Can you work these out from the model? Positions are in its coordinate system, mm. Face numbers are marked on the shaded views. A direction names the side the tool comes from. Give positions to 0.01 mm unless a question says otherwise; leave off trailing zeros. Write each loop counter-clockwise with the first axis right and the second up, starting at its lowest first coordinate (ties: lowest second). Pieces come first, ordered by that corner, then holes.
1. Suppose I cut it at B-B (y = 2.2). Please give me the cut outline in (x, z), and give its area (3 significant figures).
2. Thinking about a two-plate mould opening in Z: for the marked faces 4, 5 and 6, which applies, pulls with the +Z half, pulls with the -Z half, needs draft (parallel to the pull), parting line crosses it, or undercut?
3. On a 3-axis mill with a long thin cutter (end or side, diameter ignored), from which of +Z, -Z, +X, -X, +Y, -Y can I reach the whole of each face in a straight line? I mean the marked faces 1, 2 and 3. Say none if no direction works.
4. I'm going to push flat-ended pins straight in: pin 1 (1.3 mm diameter, centred on y = 4, z = -4, fed in from +X); pin 2 (0.6 mm diameter, centred on y = 4, z = -2, fed in from -X). Where does each tip first touch, or does it pass through?
5. Suppose I cut it at A-A (y = 3.75). Please give me the cut outline in (x, z).
6. If I drill on probe 1 along Z at (x, y) = (5, 1.3); probe 2 along Z at (x, y) = (3, 2.75); probe 3 along X at (y, z) = (1.8, -3), over which ranges is the centre line in solid material (lowest first)?
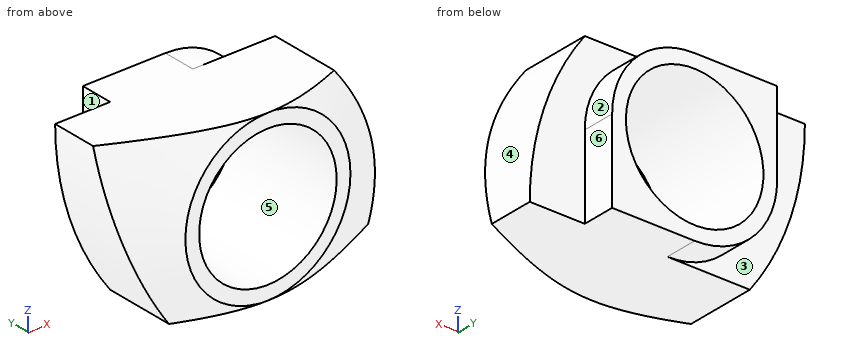
```python
from build123d import *

# Parameters (mm, degrees)
SKETCH_1_W          = 10
SKETCH_1_H          = 6
SKETCH_1_R          = 2.5
EXTRUDE_1_DEPTH     = 3.3
SKETCH_2_R          = 2.5
EXTRUDE_2_DEPTH     = 1.2
CUT_EXTRUDE_1_DEPTH = 5.5


with BuildPart() as part:
    # 草图1 → 凸台-拉伸1 (new body)
    with BuildSketch(Plane(origin=(0, 0, 0), x_dir=(1, 0, 0), z_dir=(0, 1, 0))):
        with Locations((5, 3)):
            Rectangle(SKETCH_1_W, SKETCH_1_H)
        with Locations((5, 3)):
            Circle(SKETCH_1_R, mode=Mode.SUBTRACT)
    extrude(amount=EXTRUDE_1_DEPTH)

    # 草图2 → 凸台-拉伸2 (add)
    with BuildSketch(Plane(origin=(0, 3.3, 0), x_dir=(1, 0, 0), z_dir=(0, 1, 0))):
        with BuildLine():
            Line((2, 3), (2, 0))
            Line((2, 0), (5, 0))
            ThreePointArc((5, 0), (7.121320344, 0.878679656), (8, 3))
            Line((8, 3), (8, 6))
            Line((8, 6), (5, 6))
            ThreePointArc((5, 6), (2.878679656, 5.121320344), (2, 3))
        make_face()
        with Locations((5, 3)):
            Circle(SKETCH_2_R, mode=Mode.SUBTRACT)
    extrude(amount=EXTRUDE_2_DEPTH)

    # 草图3 → 切除-拉伸1 (cut, through all)
    with BuildSketch(Plane(origin=(0, 0, 0), x_dir=(1, 0, 0), z_dir=(0, 1, 0))):
        with BuildLine():
            Line((2, 6), (0, 6))
            Line((0, 6), (0, 0))
            ThreePointArc((0, 0), (0.513167019, 3.16227766), (2, 6))
        make_face()
        with BuildLine():
            Line((10, 0), (10, 6))
            ThreePointArc((10, 6), (9.486832981, 2.83772234), (8, 0))
            Line((8, 0), (10, 0))
        make_face()
    extrude(amount=CUT_EXTRUDE_1_DEPTH, mode=Mode.SUBTRACT)

    # 草图4 one side → 切除-旋转1 (revolve, cut)
    with BuildSketch(Plane(origin=(-3, 0, -3), x_dir=(1, 0, 0), z_dir=(0, 0, 1))):
        Polygon((16, 0), (16, 2.886751346), (11, 0), align=None)
    revolve(axis=Axis((5, 3.3, -3), (0, -1, 0)), mode=Mode.SUBTRACT)


solid = part.part
```
Checks:
1. outline: (0, 0) arc R10 ccw to (2, -6) - (10, -6) arc R10 ccw to (8, 0) - close; hole circle Ø5 at (5, -3)
1. area: 32.7 mm2
2. face 4: pulls with the +Z half
2. face 5: undercut
2. face 6: needs draft
3. face 1: +Z, -Z, -X, +Y
3. face 2: +Z, +X, +Y
3. face 3: -Z, -X, +Y
4. pin 1: stops at x = 8
4. pin 2: stops at x = 2
5. outline: (2, -3) arc R3 ccw to (5, -6) - (8, -6) - (8, -3) arc R3 ccw to (5, 0) - (2, 0) - close; hole circle Ø5 at (5, -3)
6. probe 1: z = -6 to -5.5, -0.5 to 0
6. probe 2: z = -6 to -4.5, -1.5 to 0
6. probe 3: x = 0.46 to 2.5, 7.5 to 9.54
